Build history of the part. All positions in model axes, mm. A direction names the side the tool comes from. Give positions to 0.01 mm unless a question says otherwise; leave off trailing zeros. Write each loop counter-clockwise with the first axis right and the second up, starting at its lowest first coordinate (ties: lowest second). Pieces come first, ordered by that corner, then holes. Notation, with made-up numbers: (-35, 83.5) -> (-5, 83.5) arc R18 ccw to (-5, 108.5) -> close; hole circle Ø11 at (22.25, 29). An arc over 180 degrees is marked (long way). Put each result on its own line as item: value. Start each with the question number.
Item 1: Two-plate mould, pull along Z, no slides. Class faces 1 (the flat face through (-6, 0, 3)), 2 (the cylindrical face through (3.22, 8.18, 4.21)), 3 (the cylindrical face through (7.81, 2.99, 1.73)): pulls with the +Z half, pulls with the -Z half, needs draft (parallel to the pull), parting line crosses it, or undercut.
Item 2: Drill centre lines: line 1 along X through (y, z) = (8.8, 0); line 2 along Y through (x, z) = (8.25, -0.75); line 3 along Z through (x, y) = (-0.5, 2.5). Where is each one in solid material? Low to high.
Item 3: Slice it at A-A, the plane y = 9. List the corners of the cut face in (x, z).
Item 4: Tool access for faces 4 (the flat face through (7, 4, 4.3)), 5 (the cylindrical face through (9.274, 5.232, 2.059)), 6 (the flat face through (0, 12, 0)), 7 (the flat face through (0, 11, 0)), 8 (the cylindrical face through (3.955, 9.359, 5.158)): list every direction of +Z, -Z, +X, -X, +Y, -Y with a clear straight run to the whole face (end or side of a thin tool).
Item 5: Slice it at D-D, the plane y = 1.25. List the corners of the cut face in (x, z).
Item 6: Flat gauge pins, fed straight in: pin 1 Ø5.5 at (x, z) = (2, 1) entering from -Y; pin 2 Ø3 at (x, y) = (-3, 4.5) entering from -Z; pin 3 Ø2 at (x, z) = (6.5, 2) entering from +Y. Where does each tip first touch, or does it go through?
```python
from build123d import *


with BuildPart() as part:
    # Esquisse1 → Révolution1 (revolve)
    with BuildSketch(Plane.XY, mode=Mode.PRIVATE) as r_volution1_sk:
        with BuildLine():
            Line((8.345299462, 0), (6.3, 0))
            Line((6.3, 0), (5.404996879, 0.895003121))
            ThreePointArc((5.404996879, 0.895003121), (5.998873428, 3.616265174), (5.3, 6.312472222))
            Line((5.3, 6.312472222), (5.3, 10))
            ThreePointArc((5.3, 10), (5.007106781, 10.707106781), (4.3, 11))
            Line((4.3, 11), (0, 11))
            Line((0, 11), (0, 12))
            Line((0, 12), (4.5, 12))
            ThreePointArc((4.5, 12), (5.914213562, 11.414213562), (6.5, 10))
            Line((6.5, 10), (6.5, 8.736067977))
            ThreePointArc((6.5, 8.736067977), (6.526751011, 8.506315057), (6.605572809, 8.288854382))
            Line((6.605572809, 8.288854382), (7.223606798, 7.052786405))
            ThreePointArc((7.223606798, 7.052786405), (7.592302877, 6.649349192), (8.118033989, 6.5))
            Line((8.118033989, 6.5), (9.5, 6.5))
            Line((9.5, 6.5), (9.5, 4))
            Line((9.5, 4), (8, 4))
            Line((8, 4), (8, 2))
            Line((8, 2), (9.5, 2))
            Line((9.5, 2), (8.345299462, 0))
        make_face()
    revolve(r_volution1_sk.sketch.rotate(Axis((0, 0, 0), (0, 1, 0)), 90), axis=Axis((0, 0, 0), (0, 1, 0)))


solid = part.part
```
Values follow:
1. face 1: needs draft
1. face 2: undercut
1. face 3: parting line crosses it
2. line 1: -6.5 to -5.3, 5.3 to 6.5
2. line 2: 0 to 2, 4 to 6.5
2. line 3: -7.98 to -5.89, 5.89 to 7.98
3. outline: circle Ø13 at (0, 0); hole circle Ø10.6 at (0, 0)
4. face 4: none
4. face 5: +Y, -Y
4. face 6: +Z, -Z, +X, -X, +Y
4. face 7: -Y
4. face 8: +Y
5. outline: circle Ø18.13 at (0, 0); hole circle Ø11.12 at (0, 0)
6. pin 1: y = 10.73
6. pin 2: z = -9.38
6. pin 3: y = 11.52
